```python
from build123d import *

# Parameters (mm, degrees)
CYLINDER096_R     = 3
CYLINDER096_DEPTH = 3
CYLINDER095_R     = 1.7
CYLINDER095_DEPTH = 4
BOX019_W          = 24
BOX019_H          = 10
BOX019_DEPTH      = 4
BOX020_W          = 24
BOX020_H          = 10
BOX020_DEPTH      = 4
BOX021_W          = 3.6
BOX021_H          = 4
BOX021_DEPTH      = 4
CYLINDER094_R     = 11.9
CYLINDER094_DEPTH = 4
FILLET_R          = 2


with BuildPart() as obj1:
    # Cylinder096 → Cylinder096 (new body)
    with BuildSketch(Plane(origin=(0, -44, 15), x_dir=(1, 0, 0), z_dir=(0, 0, 1))):
        Circle(CYLINDER096_R)
    extrude(amount=CYLINDER096_DEPTH)


with BuildPart() as obj2:
    # Cylinder095 → Cylinder095 (new body)
    with BuildSketch(Plane(origin=(0, -44, 14), x_dir=(1, 0, 0), z_dir=(0, 0, 1))):
        Circle(CYLINDER095_R)
    extrude(amount=CYLINDER095_DEPTH)


with BuildPart() as obj3:
    # Box019 → Box019 (new body)
    with BuildSketch(Plane(origin=(-12, -37, 14), x_dir=(1, 0, 0), z_dir=(0, 0, 1))):
        with Locations((12, 5)):
            Rectangle(BOX019_W, BOX019_H)
    extrude(amount=BOX019_DEPTH)


with BuildPart() as obj4:
    # Box020 → Box020 (new body)
    with BuildSketch(Plane(origin=(9, -45, 14), x_dir=(1, 0, 0), z_dir=(0, 0, 1))):
        with Locations((12, 5)):
            Rectangle(BOX020_W, BOX020_H)
    extrude(amount=BOX020_DEPTH)


with BuildPart() as cubealignment:
    # Box021 → Box021 (new body)
    with BuildSketch(Plane(origin=(-1.8, -59, 14), x_dir=(1, 0, 0), z_dir=(0, 0, 1))):
        with Locations((1.8, 2)):
            Rectangle(BOX021_W, BOX021_H)
    extrude(amount=BOX021_DEPTH)


with BuildPart() as bearingholdertop:
    # Cylinder094 → Cylinder094 (new body)
    with BuildSketch(Plane(origin=(0, -44, 14), x_dir=(1, 0, 0), z_dir=(0, 0, 1))):
        Circle(CYLINDER094_R)
    extrude(amount=CYLINDER094_DEPTH)

    # Fusion033: union CubeAlignment
    add(cubealignment.part)

    # Cut: cut obj4
    add(obj4.part, mode=Mode.SUBTRACT)

    # Cut052: cut obj3
    add(obj3.part, mode=Mode.SUBTRACT)

    # Cut053: cut obj2
    add(obj2.part, mode=Mode.SUBTRACT)

    # Cut054: cut obj1
    add(obj1.part, mode=Mode.SUBTRACT)

    # Fillet
    fillet_edges = [bearingholdertop.edges().sort_by_distance(p)[0] for p in [
        (1.8, -55.763078, 16),
        (-1.8, -55.763078, 16),
        (11.857909, -45, 16),
        (-9.623409, -37, 16),
        (9, -37, 16),
    ]]
    fillet(fillet_edges, radius=FILLET_R)


solid = bearingholdertop.part
```
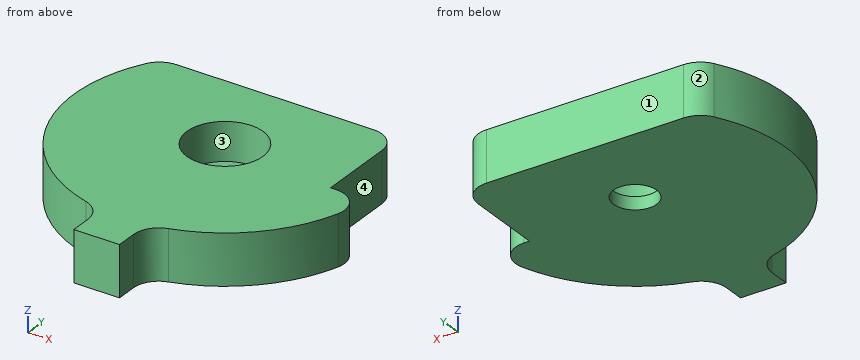
Geometry: final body of the model. Coordinates: model frame, mm. Face numbers are marked on the shaded views. Coordinates: 2 decimals unless noted, no trailing zeros. Order: outer loops, then holes, each group sorted by start corner. A loop starts at its lowest first (then second) coordinate and runs counter-clockwise, first axis right, second up. Notation, with made-up numbers: (31.25, 15.5) - (70.25, 15.5) arc R24 ccw to (70.25, 51.5) - close; hole circle Ø5 at (8, 42.5). An arc over 180 degrees is marked (long way). Return JSON: item names as keys, results as strings. Group by question number.
1. Pin query (flat end, axial travel): pin 1 (0.5 mm diameter, centred on y = -58.5, z = 16, fed in from +X); pin 2 (1.8 mm diameter, centred on y = -58.5, z = 16, fed in from -X); pin 3 (1 mm diameter, centred on y = -46.5, z = 16, fed in from -X). Return the tip coordinate at first contact, or that it passes through.
2. Material intervals for line 1 along X through (y, z) = (-44, 14.45); line 2 along Y through (x, z) = (0, 15.95); line 3 along X through (y, z) = (-44.5, 17.3), sorted ascending. Write a range as [from, to].
3. Cut plane D-D (y = -40.25). Output: boundary loops of the cut face in (x, z).
4. Cut plane C-C (x = 0). Output: boundary loops of the cut face in (y, z).
5. Cut plane A-A (y = -44). Output: boundary loops of the cut face in (x, z), plus the area to 3 significant figures.
6. Cut plane B-B (z = 14.4). Output: boundary loops of the cut face in (x, y), plus the area to 3 significant figures.
7. Pull-direction query (X, two-part tool) for the marked faces 1, 2, 3 and 4; classes: pulls with the +X half, pulls with the -X half, needs draft (parallel to the pull), parting line crosses it, or undercut.
Resolved:
{
 "1": {"pin 1": "stops at x = 1.8", "pin 2": "stops at x = -1.8", "pin 3": "stops at x = -11.73"},
 "2": {"line 1": "x = [-11.9, -1.7], [1.7, 9]", "line 2": "y = [-59, -47], [-41, -37]", "line 3": "x = [-11.89, -2.96], [2.96, 9]"},
 "3": {"outline": "(-11.29, 14) - (9, 14) - (9, 18) - (-11.29, 18) - close"},
 "4": {"outline": "(-59, 14) - (-45.7, 14) - (-45.7, 15) - (-47, 15) - (-47, 18) - (-59, 18) - close; (-42.3, 14) - (-37, 14) - (-37, 18) - (-41, 18) - (-41, 15) - (-42.3, 15) - close"},
 "5": {"outline": "(-11.9, 14) - (-1.7, 14) - (-1.7, 15) - (-3, 15) - (-3, 18) - (-11.9, 18) - close; (1.7, 14) - (9, 14) - (9, 18) - (3, 18) - (3, 15) - (1.7, 15) - close", "area": "62.2 mm²"},
 "6": {"outline": "(-10.27, -37.99) arc R11.9 ccw to (-3.25, -55.45) arc R2 cw to (-1.8, -57.37) - (-1.8, -59) - (1.8, -59) - (1.8, -57.37) arc R2 cw to (3.25, -55.45) arc R11.9 ccw to (11.34, -47.61) arc R2 ccw to (9.43, -45) - (9, -45) - (9, -39) arc R2 ccw to (7, -37) - (-8.54, -37) arc R2 ccw to start; hole circle Ø3.4 at (0, -44)", "area": "361 mm²"},
 "7": {"face 1": "needs draft", "face 2": "pulls with the -X half", "face 3": "undercut", "face 4": "pulls with the +X half"}
}
